Answer from the drawing. Dimensions are ordinates in mm from the lowest x, y and z of the part. Coordinates: 2 decimals unless noted, no trailing zeros. Loops run counter-clockwise (first coordinate to the right, second up) from the corner with the lowest first, then second, coordinate; pieces in that order, holes last. Notation, with made-up numbers: (7, 43.5) -> (53, 43.5) arc R27 cw to (53, 76.5) -> close; hole circle Ø10 at (23.5, 74). An arc over 180 degrees is marked (long way). Use a Markdown table: item, result.
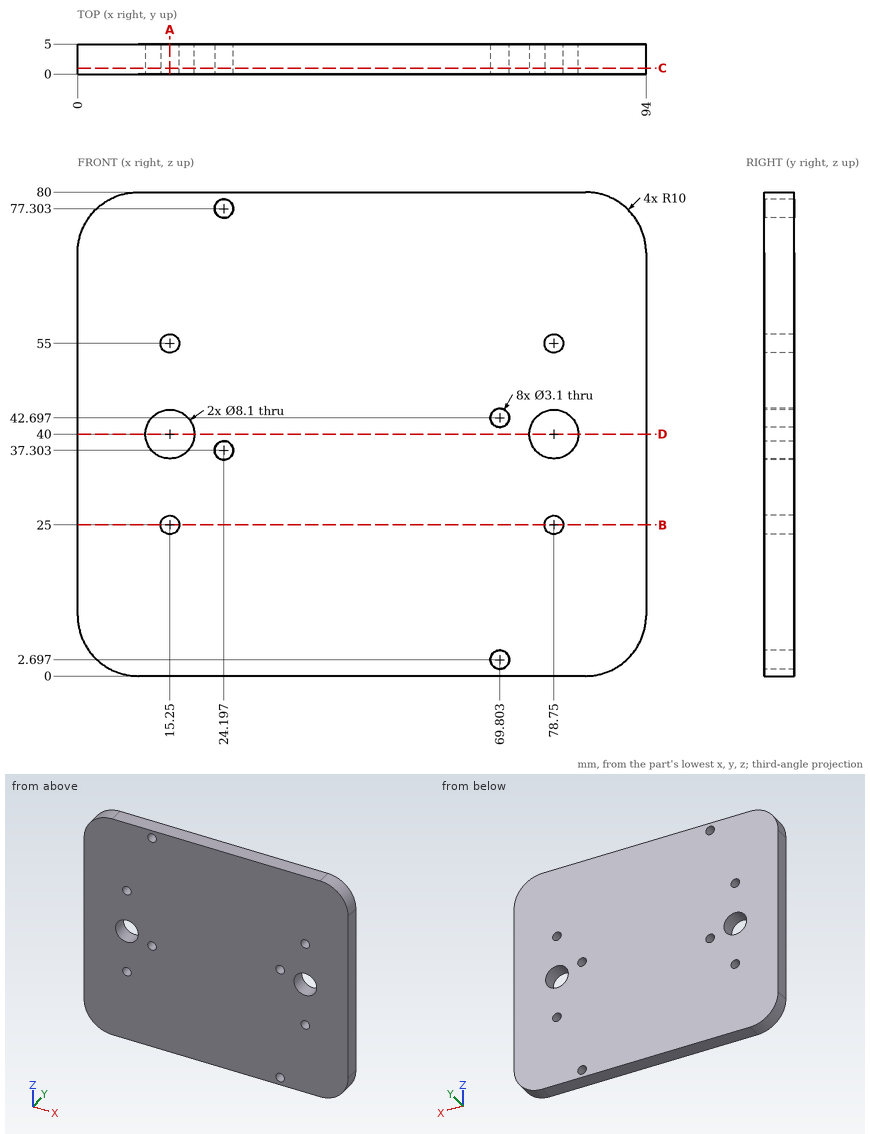
Q1. Consider line 1 (Z direction, x = 15.25, y = 2.05); line 2 (X direction, y = 1.55, z = 55); line 3 (Z direction, x = 79.5, y = 2.15). Determine where each line is inside the solid, lowest interval first. Write a range as [from, to].
Solved:
| item | result |
|---|---|
| line 1 | [0, 23.45], [26.55, 35.95], [44.05, 53.45], [56.55, 80] |
| line 2 | [0, 13.7], [16.8, 77.2], [80.3, 94] |
| line 3 | [0, 23.64], [26.36, 36.02], [43.98, 53.64], [56.36, 80] |
Q2. Section C-C on y = 1 is taken. State how many separate pieces and enclosed holes the cut face has, and give its area (3 significant figures).
Solved:
| item | result |
|---|---|
| separate pieces | 1 |
| enclosed holes | 10 |
| area | 7,270 mm² |
Q3. Given pin 1 Ø10 at (x, z) = (11, 40) entering from -Y, flat-ended and moving along its own axis, determine where the tip first touches the part or whether it passes through.
Solved:
| item | result |
|---|---|
| pin 1 | y = 0 |
Q4. Section D-D on z = 40 is taken. Determine the outline of the cut face in (x, y), and give its area (3 significant figures).
Solved:
| item | result |
|---|---|
| outline | (0, 0) -> (11.2, 0) -> (11.2, 5) -> (0, 5) -> close; (19.3, 0) -> (74.7, 0) -> (74.7, 5) -> (19.3, 5) -> close; (82.8, 0) -> (94, 0) -> (94, 5) -> (82.8, 5) -> close |
| area | 389 mm² |
Q5. Section A-A on x = 15.25 is taken. Determine the outline of the cut face in (y, z), and give its area (4 significant figures).
Solved:
| item | result |
|---|---|
| outline | (0, 0) -> (5, 0) -> (5, 23.45) -> (0, 23.45) -> close; (0, 26.55) -> (5, 26.55) -> (5, 35.95) -> (0, 35.95) -> close; (0, 44.05) -> (5, 44.05) -> (5, 53.45) -> (0, 53.45) -> close; (0, 56.55) -> (5, 56.55) -> (5, 80) -> (0, 80) -> close |
| area | 328.5 mm² |
Q6. Section B-B on z = 25 is taken. Determine the outline of the cut face in (x, y).
Solved:
| item | result |
|---|---|
| outline | (0, 0) -> (13.7, 0) -> (13.7, 5) -> (0, 5) -> close; (16.8, 0) -> (77.2, 0) -> (77.2, 5) -> (16.8, 5) -> close; (80.3, 0) -> (94, 0) -> (94, 5) -> (80.3, 5) -> close |
